from build123d import *

# Parameters (mm, degrees)
PAD_DEPTH = 4


with BuildPart() as tapered_nut_section_revolution:
    # Sketch007 → Revolution001 (revolve)
    with BuildSketch(Plane.XZ):
        Polygon((-2.5, 0), (-6.674711, 3.033105), (-5, 4), (-2.5, 4), align=None)
    revolve(axis=Axis((0, 0, 0), (0, 0, 1)))


with BuildPart() as tapered_nut_prism_section_common:
    # Sketch008 → Pad (new body)
    with BuildSketch(Plane.XY):
        Polygon((-2.886751, 5), (-5.773503, 0), (-2.886751, -5), (2.886751, -5), (5.773503, 0), (2.886751, 5), align=None)
    extrude(amount=PAD_DEPTH)

    # Common: intersect tapered-nut-section-revolution
    add(tapered_nut_section_revolution.part, mode=Mode.INTERSECT)


solid = tapered_nut_prism_section_common.part
Check sheet for the modelled part. Datum: model origin and axes. Units: mm. Give positions to 0.01 mm unless a question says otherwise; leave off trailing zeros. Write each loop counter-clockwise with the first axis right and the second up, starting at its lowest first coordinate (ties: lowest second). Pieces come first, ordered by that corner, then holes. Notation, with made-up numbers: (-1, 64) -> (6, 64) arc R17 ccw to (6, 73) -> close; hole circle Ø9 at (65.25, 46.25). An arc over 180 degrees is marked (long way). One line per item, written item: value. Start each with the question number.
Item 1: Section check B-B on z = 3.3. Record the cut outline in (x, y), then the cut area to 3 significant figures.
Item 2: Section check A-A on z = 2.1. Record the cut outline in (x, y).
Item 3: Draft check along Y on faces 1 (the flat face through (0, 5, 3)), 2 (the cylindrical face through (0.54, 2.44, 1.97)), 3 (the flat face through (2, -2, 4)). Enter one of: +Y half, -Y half, draft (parallel to the pull), parting line (faces both ways), or undercut.
Item 4: Material ranges on probe 1 along Y at (x, z) = (0, 2.95); probe 2 along Y at (x, z) = (0, 1.2); probe 3 along X at (y, z) = (-1.5, 3.65), recorded low to high. Write a range as from..to.
Item 5: Gauge pin test, flat ends, axial feed: pin 1 (3 mm diameter, centred on x = 0, y = 0, fed in from -Z); pin 2 (1 mm diameter, centred on x = -3.5, z = 3, fed in from +Y). Record the tip position at first contact, or that the pin passes through.
Results list:
1. outline: (-5.77, 0) -> (-2.89, -5) -> (2.89, -5) -> (5.77, 0) -> (2.89, 5) -> (-2.89, 5) -> close; hole circle Ø5 at (0, 0)
1. area: 67.0 mm²
2. outline: (-5.34, -0.76) -> (-3.32, -4.24) arc R5.39 ccw to (-2.01, -5) -> (2.01, -5) arc R5.39 ccw to (3.32, -4.24) -> (5.34, -0.76) arc R5.39 ccw to (5.34, 0.76) -> (3.32, 4.24) arc R5.39 ccw to (2.01, 5) -> (-2.01, 5) arc R5.39 ccw to (-3.32, 4.24) -> (-5.34, 0.76) arc R5.39 ccw to start; hole circle Ø5 at (0, 0)
3. face 1: +Y half
3. face 2: undercut
3. face 3: draft
4. probe 1: -5..-2.5, 2.5..5
4. probe 2: -4.15..-2.5, 2.5..4.15
4. probe 3: -4.91..-2, 2..4.91
5. pin 1: through
5. pin 2: y = 4.8
